CAD build for the part. Positions are in the model's coordinates, mm. A direction names the side the tool comes from. Coordinates: 2 decimals unless noted, no trailing zeros. Loops run counter-clockwise (first coordinate to the right, second up) from the corner with the lowest first, then second, coordinate; pieces in that order, holes last.
1) Wall check: line 1 along X through (y, z) = (27, -1) (3 decimals); line 2 along Y through (x, z) = (16, -3.75); line 3 along Z through (x, y) = (-68, -110). Give the ranges that are in metal, low to high.
2) Saw through at B-B, the plane x = 26. Write the cut outline in (y, z), and give its area (3 significant figures).
3) Saw through at C-C, the plane y = 4. Write the cut outline in (x, z) (1 decimal), and give its area (3 significant figures).
4) Saw through at A-A, the plane y = 88.5. Write the cut outline in (x, z) (3 decimals), and give its area (3 significant figures).
5) Two-plate mould, pull along X, no slides. Class faces 1 (the flat face through (-85.125, 53, -4)), 2 (the flat face through (83, 111.33, -4)), 3 (the flat face through (6, -108.85, -4)), 4 (the flat face through (102, -50, -7)): +X half, -X half, draft (parallel to the pull), parting line (faces both ways), or undercut.
6) Which spindle directions (+Z, -Z, +X, -X, +Y, -Y) get a long thin tool onto all of the face, cutting with end or side? Do faces 5 (the cylindrical face through (87.098, 112.344, -4.399)), 6 (the flat face through (102.539, -86, -3)), 7 (the conical face through (99.99, -109.45, 1.04)), 8 (the flat face through (102, 50, -7)), 9 (the cylindrical face through (-80.397, -1.524, -5.685)). Say none if no direction does.
7) Pin check, flat tips, straight feed: pin 1 Ø1.8 at (x, z) = (95, -7.5) entering from +Y; pin 2 Ø0.5 at (x, z) = (95, -7.5) entering from -Y; pin 3 Ø4 at (x, z) = (84.8, -4.5) entering from +Y. Stop position of each tip, or through.
```python
from build123d import *

# Parameters (mm, degrees)
PAD004_DEPTH      = 1.2
PAD004_DEPTH_BACK = 9
SKETCH007_W       = 175.4
SKETCH007_H       = 217.7
POCKET001_DEPTH   = 19
PAD005_DEPTH      = 110
POCKET002_DEPTH   = 50
POCKET003_DEPTH   = 69.5
POCKET004_DEPTH   = 17
POCKET005_DEPTH   = 9.2
SKETCH034_R       = 2.3
POCKET023_DEPTH   = 2
SKETCH035_R       = 1.25
POCKET024_DEPTH   = 16
SKETCH037_R       = 2.3
POCKET026_DEPTH   = 2
SKETCH038_R       = 1.3
POCKET027_DEPTH   = 20
CHAMFER002_SIZE   = 1
HOLE_D            = 2.7
HOLE_DEPTH        = 25
HOLE_CBORE_D      = 4.6
HOLE_CBORE_DEPTH  = 2
HOLE_TIPS_R       = 1.35
SKETCH058_W       = 4.368927
SKETCH058_H       = 1.6
POCKET037_DEPTH   = 3


with BuildPart() as part:
    # Sketch006 → Pad004 (new body, two sides)
    with BuildSketch(Plane.XY) as pad004_sk:
        with BuildLine():
            ThreePointArc((-75.625, 113.33), (-83.756728, 109.961728), (-87.125, 101.83))
            Line((-87.125, -101.83), (-87.125, 101.83))
            ThreePointArc((-87.125, -101.83), (-83.756728, -109.961728), (-75.625, -113.33))
            Line((92.538879, -113.33), (-75.625, -113.33))
            ThreePointArc((92.538879, -113.33), (100.670607, -109.961728), (104.038879, -101.83))
            Line((104.038879, 101.83), (104.038879, -101.83))
            ThreePointArc((104.038879, 101.83), (100.670607, 109.961728), (92.538879, 113.33))
            Line((-75.625, 113.33), (92.538879, 113.33))
        make_face()
        with BuildLine():
            ThreePointArc((-75.625, 104.33), (-77.392767, 103.597767), (-78.125, 101.83))
            Line((-78.125, -101.83), (-78.125, 101.83))
            ThreePointArc((-78.125, -101.83), (-77.392767, -103.597767), (-75.625, -104.33))
            Line((75.625, -104.33), (-75.625, -104.33))
            ThreePointArc((75.625, -104.33), (77.392767, -103.597767), (78.125, -101.83))
            Line((78.125, 101.83), (78.125, -101.83))
            ThreePointArc((78.125, 101.83), (77.392767, 103.597767), (75.625, 104.33))
            Line((-75.625, 104.33), (75.625, 104.33))
        make_face(mode=Mode.SUBTRACT)
    extrude(amount=PAD004_DEPTH)
    extrude(pad004_sk.sketch, amount=-PAD004_DEPTH_BACK)

    # Sketch007 → Pocket001 (cut)
    with BuildSketch(Plane(origin=(0, 0, 0), x_dir=(-1, 0, 0), z_dir=(0, 0, -1))):
        with Locations((-5.066844, 0)):
            Rectangle(SKETCH007_W, SKETCH007_H)
    extrude(amount=POCKET001_DEPTH, mode=Mode.SUBTRACT)

    # Sketch008 → Pad005 (join, symmetric)
    with BuildSketch(Plane.XZ):
        with BuildLine():
            ThreePointArc((-79.625, -9), (-80.634367, -5.242118), (-83.390781, -2.495724))
            Line((-83.390781, -2.495724), (-83.390781, -9))
            Line((-79.625, -9), (-83.390781, -9))
        make_face()
    extrude(amount=PAD005_DEPTH, both=True)

    # Sketch009 → Pocket002 (cut, symmetric)
    with BuildSketch(Plane.XZ):
        with BuildLine():
            ThreePointArc((-82.125, -9), (-83.589466, -5.464466), (-87.125, -4))
            Line((-87.125, -9), (-87.125, -4))
            Line((-82.125, -9), (-87.125, -9))
        make_face()
        with BuildLine():
            ThreePointArc((104.038879, -4), (100.503345, -5.464466), (99.038879, -9))
            Line((99.038879, -9), (104.038879, -9))
            Line((104.038879, -9), (104.038879, -4))
        make_face()
    extrude(amount=POCKET002_DEPTH, both=True, mode=Mode.SUBTRACT)

    # Sketch010 → Pocket003 (cut, symmetric)
    with BuildSketch(Plane.XZ):
        with BuildLine():
            Line((92.766844, 0), (96.966844, 0))
            ThreePointArc((93.766844, -9), (96.143042, -4.775982), (96.966844, 0))
            Line((92.766844, -9), (93.766844, -9))
            Line((92.766844, -8), (92.766844, -9))
            Line((92.766844, -8), (92.766844, 0))
        make_face()
    extrude(amount=POCKET003_DEPTH, both=True, mode=Mode.SUBTRACT)

    # Sketch011 (on DatumPlane) → Pocket004 (cut)
    with BuildSketch(Plane.YZ.offset(104.038879)):
        with BuildLine():
            ThreePointArc((-93.025352, -3.338275), (-94.925352, -5.238275), (-93.025352, -7.138275))
            Line((-93.025352, -7.138275), (-86.925352, -7.138275))
            ThreePointArc((-86.925352, -7.138275), (-85.025352, -5.238275), (-86.925352, -3.338275))
            Line((-86.925352, -3.338275), (-93.025352, -3.338275))
        make_face()
    extrude(amount=-POCKET004_DEPTH, mode=Mode.SUBTRACT)

    # Sketch012 (on DatumPlane) → Pocket005 (cut)
    with BuildSketch(Plane(origin=(0, 0, -9.2), x_dir=(1, 0, 0), z_dir=(0, 0, -1))):
        with BuildLine():
            ThreePointArc((102.538879, 99.723724), (102.099539, 100.784384), (101.038879, 101.223724))
            Line((49.822763, 101.223724), (101.038879, 101.223724))
            ThreePointArc((49.822763, 101.223724), (48.762103, 100.784384), (48.322763, 99.723724))
            Line((48.322763, 72.43325), (48.322763, 99.723724))
            ThreePointArc((48.322763, 72.43325), (48.762103, 71.37259), (49.822763, 70.93325))
            Line((101.038879, 70.93325), (49.822763, 70.93325))
            ThreePointArc((101.038879, 70.93325), (102.099539, 71.37259), (102.538879, 72.43325))
            Line((102.538879, 99.723724), (102.538879, 72.43325))
        make_face()
    extrude(amount=-POCKET005_DEPTH, mode=Mode.SUBTRACT)

    # Sketch034 (on DatumPlane) → Pocket023 (cut)
    with BuildSketch(Plane.XZ.offset(113.33)):
        with Locations((-68.2, -4.5)):
            Circle(SKETCH034_R)
        with Locations((84.8, -4.5)):
            Circle(SKETCH034_R)
    extrude(amount=-POCKET023_DEPTH, mode=Mode.SUBTRACT)

    # Sketch035 (on DatumPlane) → Pocket024 (cut)
    with BuildSketch(Plane.XZ.offset(113.33)):
        with Locations((84.8, -4.5)):
            Circle(SKETCH035_R)
        with Locations((-68.2, -4.5)):
            Circle(SKETCH035_R)
    extrude(amount=-POCKET024_DEPTH, mode=Mode.SUBTRACT)

    # Sketch037 (on DatumPlane) → Pocket026 (cut)
    with BuildSketch(Plane(origin=(0, 113.33, 0), x_dir=(-1, 0, 0), z_dir=(0, 1, 0))):
        with Locations((-84.8, -4.5)):
            Circle(SKETCH037_R)
        with Locations((68.2, -4.5)):
            Circle(SKETCH037_R)
    extrude(amount=-POCKET026_DEPTH, mode=Mode.SUBTRACT)

    # Sketch038 (on DatumPlane) → Pocket027 (cut)
    with BuildSketch(Plane(origin=(0, 113.33, 0), x_dir=(-1, 0, 0), z_dir=(0, 1, 0))):
        with Locations((-84.8, -4.5)):
            Circle(SKETCH038_R)
        with Locations((68.2, -4.5)):
            Circle(SKETCH038_R)
    extrude(amount=-POCKET027_DEPTH, mode=Mode.SUBTRACT)

    # Chamfer002
    chamfer002_edges = [part.edges().sort_by_distance(p)[0] for p in [
        (100.670607, 109.961728, 1.2),
    ]]
    chamfer(chamfer002_edges, length=CHAMFER002_SIZE)

    # Hole
    with Locations(Plane(origin=(-87.125, 0, 0), x_dir=(0, -1, 0), z_dir=(-1, 0, 0))):
        with Locations((-54.5, -4.5), (54.5, -4.5)):
            CounterBoreHole(HOLE_D / 2, HOLE_CBORE_D / 2, HOLE_CBORE_DEPTH, depth=HOLE_DEPTH)

    # Hole tips → Hole tip 1 section 0
    with BuildSketch(Plane(origin=(-62.125, 0, 0), x_dir=(0, -1, 0), z_dir=(-1, 0, 0)), mode=Mode.PRIVATE) as hole_tip_1_s0:
        with Locations((-54.5, -4.5)):
            Circle(HOLE_TIPS_R)
    loft([hole_tip_1_s0.sketch, Vertex(-61.313838, 54.5, -4.5)], mode=Mode.SUBTRACT)

    # Hole tips → Hole tip 2 section 0
    with BuildSketch(Plane(origin=(-62.125, 0, 0), x_dir=(0, -1, 0), z_dir=(-1, 0, 0)), mode=Mode.PRIVATE) as hole_tip_2_s0:
        with Locations((54.5, -4.5)):
            Circle(HOLE_TIPS_R)
    loft([hole_tip_2_s0.sketch, Vertex(-61.313838, -54.5, -4.5)], mode=Mode.SUBTRACT)

    # Sketch058 → Pocket037 (cut, symmetric)
    with BuildSketch(Plane.XZ.offset(12)):
        with Locations((94.184463, -7.2)):
            Rectangle(SKETCH058_W, SKETCH058_H)
    pocket037 = extrude(amount=POCKET037_DEPTH, both=True, mode=Mode.SUBTRACT)

    # Mirrored: Pocket037 across XZ
    add(pocket037.mirror(Plane.XZ), mode=Mode.SUBTRACT)


solid = part.part
```
Data:
1. line 1: x = -87.125 to -82.633, 96.932 to 104.039
1. line 2: y = -113.33 to -108.85, 108.85 to 113.33
1. line 3: z = -9 to -5.73, -3.27 to 1.2
2. outline: (-113.33, -9) - (-108.85, -9) - (-108.85, 0) - (-104.33, 0) - (-104.33, 1.2) - (-112.33, 1.2) - (-113.33, 0.2) - close; (104.33, 0) - (108.85, 0) - (108.85, -9) - (113.33, -9) - (113.33, 0.2) - (112.33, 1.2) - (104.33, 1.2) - close
2. area: 101 mm2
3. outline: (-87.1, -4) arc R5 cw to (-82.1, -9) - (-79.6, -9) arc R7.5 ccw to (-82.6, -3) - (-82.6, 0) - (-78.1, 0) - (-78.1, 1.2) - (-86.1, 1.2) - (-87.1, 0.2) - close; (78.1, 0) - (97, 0) arc R14.3 cw to (93.8, -9) - (99, -9) arc R5 cw to (104, -4) - (104, 0.2) - (103, 1.2) - (78.1, 1.2) - close
3. area: 127 mm2
4. outline: (-87.125, -9) - (-79.625, -9) arc R7.5 ccw to (-82.633, -2.994) - (-82.633, 0) - (-78.125, 0) - (-78.125, 1.2) - (-86.125, 1.2) - (-87.125, 0.2) - close; (78.125, 0) - (92.767, 0) - (92.767, -9) - (104.039, -9) - (104.039, 0.2) - (103.039, 1.2) - (78.125, 1.2) - close
4. area: 195 mm2
5. face 1: -X half
5. face 2: undercut
5. face 3: undercut
5. face 4: draft
6. face 5: +Y
6. face 6: -Z
6. face 7: +Z, +X, -Y
6. face 8: -Z, +X
6. face 9: none
7. pin 1: stops at y = 113.22
7. pin 2: stops at y = -113.12
7. pin 3: stops at y = 111.33
